Autodesk Inventor part; units mm, degrees
ref_plane "YZ Plane" through (0, 0, 0) normal (1, 0, 0) x (0, 1, 0)
ref_plane "XZ Plane" through (0, 0, 0) normal (0, 1, 0) x (-1, 0, 0)
ref_plane "XY Plane" through (0, 0, 0) normal (0, 0, 1) x (1, 0, 0)
sketch "Sketch1" plane through (0, 0, 0) normal (0, 1, 0) x (-1, 0, 0)
  circle A0 centre (-7.5, 8.25) radius 0.875
  circle A1 centre (-7.5, -8.25) radius 0.875
  circle A2 centre (33.5, 8.25) radius 0.875
  circle A3 centre (33.5, -8.25) radius 0.875
  circle A4 centre (0, 0) radius 8.6279
  circle A5 centre (26, 0) radius 8.6279
  line L0 (-13.5, -14) -> (36.5, -14)
  line L1 (39.5, 45) -> (21.5, 45)
  line L2 (21.5, 45) -> (21.5, 37)
  line L3 (4.5, 45) -> (4.5, 37)
  line L4 (19.5, 35) -> (6.5, 35)
  line L5 (39.5, 45) -> (21.5, 45)
  line L6 (4.5, 45) -> (-13.5, 45)
  line L7 (-13.5, 45) -> (39.285, 45) construction
  arc A6 (19.5, 35) -> (21.5, 37) centre (19.5, 37) ccw
  arc A7 (4.5, 37) -> (6.5, 35) centre (6.5, 37) ccw
  line L8 (-10.5, -14) -> (-10.5, 1)
  line L9 (-10.5, 1) -> (-13.5, 1)
  line L10 (-13.5, 1) -> (-13.5, 16)
  line L11 (-13.5, 16) -> (-10.5, 16)
  line L12 (-10.5, 16) -> (-10.5, 31)
  line L13 (-10.5, 31) -> (-13.5, 31)
  line L14 (-13.5, 45) -> (-13.5, 31)
  line L15 (-13.5, 16) -> (-13.5, 1)
  line L16 (36.5, -14) -> (36.5, 1)
  line L17 (36.5, 1) -> (39.5, 1)
  line L18 (39.5, 16) -> (36.5, 16)
  line L19 (36.5, 16) -> (36.5, 31)
  line L20 (36.5, 31) -> (39.5, 31)
  line L21 (39.5, 1) -> (39.5, 16)
  line L22 (39.5, 31) -> (39.5, 45)
  point P0 (35.5, -10)
  point P1 (21.5, 35)
  dimension "d5" = 1.75
  dimension "d6" = 1.75
  dimension "d7" = 1.75
  dimension "d8" = 1.75
  dimension "d11" = 18
  dimension "d12" = 10
  dimension "d14" = 2
  dimension "d15" = 3
  dimension "d17" = 15
  dimension "d18" = 15
extrude "Extrusion1" add sketch "Sketch1" along normal blind 3
properties part number "do_sensor_1_3mm"
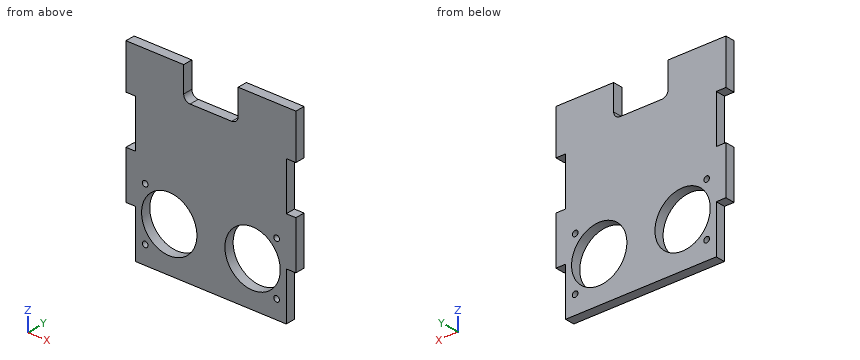
Input: part model. Units: mm. Frame: model coordinates. Give positions to 0.01 mm unless a question says otherwise; leave off trailing zeros. Loops run counter-clockwise (first coordinate to the right, second up) from the corner with the lowest first, then second, coordinate; pieces in that order, holes last.
1) Contact query for flat-ended pins moving along their axis: pin 1 (1.4 mm diameter, centred on x = 7.5, z = 8.25, fed in from +Y); pin 2 (1.5 mm diameter, centred on y = 1.5, z = 21, fed in from +X); pin 3 (0.9 mm diameter, centred on y = 2, z = -6, fed in from -X); pin 4 (0.9 mm diameter, centred on x = 12, y = 1.5, fed in from -Z). Output: stop coordinate, or through.
A:
pin 1: passes through
pin 2: stops at x = 10.5
pin 3: stops at x = -36.5
pin 4: stops at z = 1
2) Section query D-D on z = 41. Return the cut outline in (x, y).
A:
outline: (-39.5, 0) - (-21.5, 0) - (-21.5, 3) - (-39.5, 3) - close; (-4.5, 0) - (13.5, 0) - (13.5, 3) - (-4.5, 3) - close
3) Section query A-A on x = -26. Return the cut outline in (y, z).
A:
outline: (0, -14) - (3, -14) - (3, -8.63) - (0, -8.63) - close; (0, 8.63) - (3, 8.63) - (3, 45) - (0, 45) - close
4) Section query B-B on z = 0. Return the cut outline in (x, y).
A:
outline: (-36.5, 0) - (-34.63, 0) - (-34.63, 3) - (-36.5, 3) - close; (-17.37, 0) - (-8.63, 0) - (-8.63, 3) - (-17.37, 3) - close; (8.63, 0) - (10.5, 0) - (10.5, 3) - (8.63, 3) - close
5) Line query: L1, parallel to X at y = 0.6, z = -1; L2, parallel to Z at x = 0, y = 1.2; L3, parallel to Z at x = -33.5, y = 1.65 (3 decimals). Output: solid intervals per line, ascending.
A:
L1: x = -36.5 to -34.57, -17.43 to -8.57, 8.57 to 10.5
L2: z = -14 to -8.63, 8.63 to 45
L3: z = -14 to -9.125, -7.375 to -4.265, 4.265 to 7.375, 9.125 to 45
6) Section query C-C on y = 2.25. Return the cut outline in (x, z) (3 decimals), and give its area (3 significant figures).
A:
outline: (-39.5, 1) - (-36.5, 1) - (-36.5, -14) - (10.5, -14) - (10.5, 1) - (13.5, 1) - (13.5, 16) - (10.5, 16) - (10.5, 31) - (13.5, 31) - (13.5, 45) - (-4.5, 45) - (-4.5, 37) arc R2 cw to (-6.5, 35) - (-19.5, 35) arc R2 cw to (-21.5, 37) - (-21.5, 45) - (-39.5, 45) - (-39.5, 31) - (-36.5, 31) - (-36.5, 16) - (-39.5, 16) - close; hole circle Ø17.256 at (-26, 0); hole circle Ø1.75 at (-33.5, -8.25); hole circle Ø1.75 at (-33.5, 8.25); hole circle Ø17.256 at (0, 0); hole circle Ø1.75 at (7.5, -8.25); hole circle Ø1.75 at (7.5, 8.25)
area: 2,300 mm2
